Autodesk Inventor part; units mm, degrees
ref_plane "Work Plane1" through (0, 0, -9.398) normal (0, 0, 1) x (1, 0, 0)
ref_plane "Work Plane6" through (0, 13.462, 0) normal (0, 1, 0) x (-1, 0, 0)
ref_plane "Work Plane7" through (0, 0, 8.128) normal (0, 0, 1) x (1, 0, 0)
sketch "Sketch2" plane through (0, 0, 0) normal (0, 0, 1) x (1, 0, 0)
  circle A0 centre (0, 0) radius 8.382
  dimension "d0" = 16.764
extrude "Extrusion1" add sketch "Sketch2" along normal blind 13.97
sketch "Sketch3" plane through (0, 0, 0) normal (0, 0, -1) x (-1, 0, 0)
  circle A0 centre (0, 0) radius 8.382
  circle A1 centre (0, 0) radius 8.89
  dimension "d3" = 17.78
extrude "Extrusion2" add sketch "Sketch3" along normal blind 17.018 contours A0 | A1
ref_plane "Work Plane1" through (0, 0, -9.398) normal (0, 0, 1) x (1, 0, 0)
sketch "Sketch4" plane through (0, 0, -9.398) normal (0, 0, 1) x (1, 0, 0)
  circle A0 centre (0, 0) radius 8.89
  circle A1 centre (0, 0) radius 10.287
  circle A2 centre (0, 0) radius 8.89
  dimension "d7" = 20.574
extrude "Extrusion3" add sketch "Sketch4" against normal blind 2.54
ref_plane "Work Plane6" through (0, 13.462, 0) normal (0, 1, 0) x (-1, 0, 0)
ref_plane "Work Plane5" through (0, 8.89, 0) normal (0, 1, 0) x (-1, 0, 0)
sketch "Sketch6" plane through (0, 13.462, 0) normal (0, 1, 0) x (-1, 0, 0)
  circle A0 centre (0, -10.668) radius 3.937
  line L0 (-9.4933, -9.398) -> (9.4933, -9.398)
  line L1 (9.4933, -11.938) -> (-9.4933, -11.938)
  line L2 (0, -24.5018) -> (0, -30.8914) construction
  point P0 (0, 0)
  dimension "d16" = 7.874
  dimension "d17" = 1.27
extrude "Extrusion4" add sketch "Sketch6" against normal up to surface
ref_plane "Work Plane7" through (0, 0, 8.128) normal (0, 0, 1) x (1, 0, 0)
sketch "Sketch7" plane through (0, 0, 8.128) normal (0, 0, 1) x (1, 0, 0)
  circle A0 centre (0, 0) radius 8.382
  line L0 (-1.905, 8.1627) -> (-1.905, 11.2107)
  line L1 (-1.905, 11.2107) -> (1.905, 11.2107)
  line L2 (1.905, 11.2107) -> (1.905, 8.1627)
  arc A1 (1.905, 8.1627) -> (-1.905, 8.1627) centre (0, 0) ccw
  dimension "d25" = 16.764
  dimension "d26" = 3.81
  dimension "d27" = 3.048
  dimension "d28" = 1.905
extrude "Extrusion5" add sketch "Sketch7" against normal up to surface contours A0 L0 L1 L2
pattern_circular "Circular Pattern1" count 2 over 360 about axis through (0, 0, 0) along (0, 0, 1) of "Extrusion4", "Extrusion5"
sketch "Sketch8" plane through (0, 13.462, -10.668) normal (0, 1, 0) x (1, 0, 0)
  circle A0 centre (0, 0) radius 3.937
  circle A1 centre (0, 0) radius 1.27
  point P0 (0, -10.668)
  dimension "d34" = 2.54
extrude "Extrusion6" add sketch "Sketch8" along normal blind 9.525 contours A1
pattern_circular "Circular Pattern2" count 2 over 360 about axis through (0, 0, 0) along (0, 0, 1) of "Extrusion6"
sketch "Sketch9" plane through (0, 0, -17.018) normal (0, 0, -1) x (-1, 0, 0)
  circle A0 centre (0, 0) radius 8.89
  circle A1 centre (0, 0) radius 6.985
  dimension "d40" = 13.97
extrude "Extrusion7" cut sketch "Sketch9" against normal blind 28.448 contours A1
sketch "Sketch10" plane through (0, 0, 13.97) normal (0, 0, 1) x (1, 0, 0)
  circle A0 centre (0, 0) radius 8.382
  circle A1 centre (0, 0) radius 4.445
  dimension "d43" = 8.89
extrude "Extrusion8" cut sketch "Sketch10" against normal up to surface (2.54 mm away) contours A1
sketch "Sketch12" plane through (0, 0, 0) normal (0, 1, 0) x (-1, 0, 0)
  line L0 (-10.287, -17.018) -> (-10.287, 2.032)
  circle A0 centre (-18.4993, -17.2721) radius 1.27
  arc A1 (-20.699, -16.0021) -> (-17.6397, -19.6623) centre (-18.4993, -17.2721) ccw
  line L1 (-10.287, 2.032) -> (-20.699, -16.0021)
  line L2 (-10.287, -17.018) -> (-17.6397, -19.6623)
  line L3 (8.89, -17.018) -> (-8.89, -17.018)
  line L4 (-10.287, -9.398) -> (-10.287, -11.938)
  line L5 (0, -20.2977) -> (0, -33.1857) construction
  line L6 (10.287, -17.018) -> (10.287, 2.032)
  circle A2 centre (18.4993, -17.2721) radius 1.27
  arc A3 (17.6397, -19.6623) -> (20.699, -16.0021) centre (18.4993, -17.2721) ccw
  line L7 (10.287, 2.032) -> (20.699, -16.0021)
  line L8 (10.287, -17.018) -> (17.6397, -19.6623)
  line L9 (10.287, -9.398) -> (10.287, -11.938)
  point P0 (0, 0)
  dimension "d46" = 2.54
  dimension "d47" = 5.08
  dimension "d48" = 30
  dimension "d49" = 19.05
extrude "Extrusion9" add sketch "Sketch12" along normal mid plane 2.54
sketch "Sketch13" plane through (10.287, -1.27, -17.018) normal (-1, 0, 0) x (0, 0, 1)
  line L0 (0, 2.54) -> (19.05, 2.54)
  line L1 (19.05, 2.54) -> (19.05, 0)
  line L2 (19.05, 0) -> (0, 0)
  line L3 (0, 0) -> (0, 2.54)
  point P0 (17.018, 1.27)
extrude "Extrusion10" add sketch "Sketch13" along normal up to surface
mirror "Mirror1" about plane through (0, 0, 0) normal (1, 0, 0) of "Extrusion10"
properties part number "Axle Body - Front - Custom"
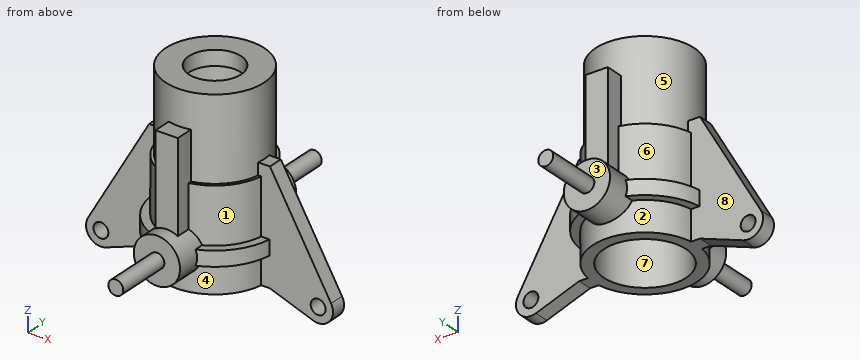
Source: CAD feature listing. Evaluate the final solid. Frame: model axes, mm. Face numbers are marked on the shaded views. A direction names the side the tool comes from. Coordinates: 2 decimals unless noted, no trailing zeros. Write each loop counter-clockwise with the first axis right and the second up, starting at its lowest first coordinate (ties: lowest second). Pieces come first, ordered by that corner, then holes. Notation, with made-up numbers: (-25.75, 22) - (0.25, 22) arc R13 cw to (0.25, 46) - close; hole circle Ø3 at (40, 87.25). An arc over 180 degrees is marked (long way). Answer as a JSON object with one key per item and string values.
Q1. Section query C-C, the plane y = 0. Output: boundary loops of the cut face in (x, z) (3 decimals), plus the area to 3 significant figures.
Ans:
{"outline": "(-20.699, -16.002) arc R2.54 ccw to (-17.64, -19.662) - (-10.287, -17.018) - (-6.985, -17.018) - (-6.985, 11.43) - (-4.445, 11.43) - (-4.445, 13.97) - (-8.382, 13.97) - (-8.382, 2.032) - (-10.287, 2.032) - close; (4.445, 11.43) - (6.985, 11.43) - (6.985, -17.018) - (10.287, -17.018) - (17.64, -19.662) arc R2.54 ccw to (20.699, -16.002) - (10.287, 2.032) - (8.382, 2.032) - (8.382, 13.97) - (4.445, 13.97) - close; hole circle Ø2.54 at (-18.499, -17.272); hole circle Ø2.54 at (18.499, -17.272)", "area": "407 mm2"}
Q2. Section query A-A, the plane z = 3. Output: boundary loops of the cut face in (x, y) (3 decimals).
Ans:
{"outline": "(-1.905, -11.211) - (1.905, -11.211) - (1.905, -8.163) arc R8.382 ccw to (1.905, 8.163) - (1.905, 11.211) - (-1.905, 11.211) - (-1.905, 8.163) arc R8.382 ccw to (-1.905, -8.163) - close; hole circle Ø13.97 at (0, 0)"}
Q3. Material intervals for line 1 (Z direction, x = -6, y = -3); line 2 (Y direction, x = 4.5, z = 6.5); line 3 (Y direction, x = -2.5, z = 11), sorted ascending. Write a range as [from, to].
Ans:
{"line 1": "z = [11.43, 13.97]", "line 2": "y = [-7.07, -5.34], [5.34, 7.07]", "line 3": "y = [-8, -6.52], [6.52, 8]"}
Q4. First-contact query: pin 1 Ø2.5 at (x, y) = (0.5, -10.5) entering from +Z; pin 2 Ø4 at (x, z) = (-10, -12.5) entering from -Y; pin 3 Ø4 at (x, z) = (14.5, -12.5) entering from +Y. Flat tips, straight axial feed; report the tip coordinate or a pass-through.
Ans:
{"pin 1": "stops at z = 8.13", "pin 2": "stops at y = -6.37", "pin 3": "stops at y = 1.27"}
Q5. Draft query along X for the marked faces 6, 7 and 8. Return one class per face: released by +X, released by -X, zero draft, split by the parting line, or undercut.
Ans:
{"face 6": "released by -X", "face 7": "undercut", "face 8": "zero draft"}
Q6. Set-up query: the marked faces 1, 2, 3, 4 and 5. Return all of +Z, -Z, +X, -X, +Y, -Y with unobstructed straight access to the full face (end or side cutting, diameter ignored); none if empty.
Ans:
{"face 1": "+Z, +X, -Y", "face 2": "-Z, +Y", "face 3": "+Y", "face 4": "-Z, -Y", "face 5": "+Z"}
Q7. Section query D-D, the plane x = 6. Output: boundary loops of the cut face in (y, z).
Ans:
{"outline": "(-8.36, -11.94) - (-6.56, -11.94) - (-6.56, -17.02) - (-3.58, -17.02) - (-3.58, 11.43) - (3.58, 11.43) - (3.58, -17.02) - (6.56, -17.02) - (6.56, -11.94) - (8.36, -11.94) - (8.36, -9.4) - (6.56, -9.4) - (6.56, 0) - (5.85, 0) - (5.85, 13.97) - (-5.85, 13.97) - (-5.85, 0) - (-6.56, 0) - (-6.56, -9.4) - (-8.36, -9.4) - close"}
